from build123d import *

# Parameters (mm, degrees)
ESQUISSE1_W             = 8
ESQUISSE1_H             = 20
BOSS_EXTRU_1_DEPTH      = 12
ESQUISSE2_W             = 8
ESQUISSE2_H             = 10
ENL_V_MAT_EXTRU_1_DEPTH = 8
ESQUISSE3_R             = 3
ENL_V_MAT_EXTRU_2_DEPTH = 10
ESQUISSE4_R             = 3
ENL_V_MAT_EXTRU_3_DEPTH = 4


with BuildPart() as part:
    # Esquisse1 → Boss.-Extru.1 (new body)
    with BuildSketch(Plane.XY):
        Rectangle(ESQUISSE1_W, ESQUISSE1_H)
    extrude(amount=BOSS_EXTRU_1_DEPTH)

    # Esquisse2 → Enlèv. mat.-Extru.1 (cut)
    with BuildSketch(Plane.ZY.offset(4)):
        with Locations((8, -5)):
            Rectangle(ESQUISSE2_W, ESQUISSE2_H)
    extrude(amount=-ENL_V_MAT_EXTRU_1_DEPTH, mode=Mode.SUBTRACT)

    # Esquisse3 → Enlèv. mat.-Extru.2 (cut)
    with BuildSketch(Plane.XZ):
        with Locations(Location((0, 8, 0), (0, 0, 270))):
            Circle(ESQUISSE3_R)
    extrude(amount=-ENL_V_MAT_EXTRU_2_DEPTH, mode=Mode.SUBTRACT)

    # Esquisse4 → Enlèv. mat.-Extru.3 (cut)
    with BuildSketch(Plane.XY.offset(4)):
        with Locations((0, -5)):
            Circle(ESQUISSE4_R)
    extrude(amount=-ENL_V_MAT_EXTRU_3_DEPTH, mode=Mode.SUBTRACT)


solid = part.part
Model file for the job. Use its own axes, mm. A direction names the side the tool comes from. Give positions to 0.01 mm unless a question says otherwise; leave off trailing zeros. Order: outer loops, then holes, each group sorted by start corner. A loop starts at its lowest first (then second) coordinate and runs counter-clockwise, first axis right, second up. Notation, with made-up numbers: (-6.75, 39) - (31.25, 39) arc R23 cw to (31.25, 60) - close; hole circle Ø8 at (58, 84.5). An arc over 180 degrees is marked (long way). One line per item, written item: value.
Item 1: Pin check, flat tips, straight feed: pin 1 Ø4 at (y, z) = (-3.5, 4.5) entering from +X; pin 2 Ø2 at (x, y) = (3, -5.5) entering from +Z. Stop position of each tip, or through.
Response values:
pin 1: x = 4
pin 2: z = 4
Item 2: Slice it at A-A (z = 8). List the corners of the cut face in (x, y).
Response values:
outline: (-4, 0) - (-3, 0) - (-3, 10) - (-4, 10) - close; (3, 0) - (4, 0) - (4, 10) - (3, 10) - close
Item 3: Wall check: line 1 (X direction, y = 4, z = 8); line 2 (Y direction, x = 3, z = 10); line 3 (Y direction, x = 0, z = 0.9). Give the ranges that are in metal, low to high.
Response values:
line 1: -4 to -3, 3 to 4
line 2: 0 to 10
line 3: -10 to -8, -2 to 10
Item 4: Slice it at C-C (x = 0). List the corners of the cut face in (y, z).
Response values:
outline: (-10, 0) - (-8, 0) - (-8, 4) - (-10, 4) - close; (-2, 0) - (10, 0) - (10, 5) - (0, 5) - (0, 4) - (-2, 4) - close; (0, 11) - (10, 11) - (10, 12) - (0, 12) - close
Item 5: Tool access for faces 1 (the flat face through (-3, 0, 10)), 2 (the flat face through (-0.1, 10, 4.6)): list every direction of +Z, -Z, +X, -X, +Y, -Y with a clear straight run to the whole face (end or side of a thin tool).
Response values:
face 1: +Z, +X, -X, -Y
face 2: +Z, -Z, +X, -X, +Y
Item 6: Slice it at B-B (y = -5). List the corners of the cut face in (x, z), then the cut area to 3 significant figures.
Response values:
outline: (-4, 0) - (-3, 0) - (-3, 4) - (-4, 4) - close; (3, 0) - (4, 0) - (4, 4) - (3, 4) - close
area: 8.00 mm2
Item 7: Two-plate mould, pull along Y, no slides. Class faces 3 (the flat face through (0, -10, 2)), 4 (the cylindrical face through (0.9, 4.93, 5.14)), 5 (the cylindrical face through (0, -2, 2)): released by +Y, released by -Y, zero draft, split by the parting line, or undercut.
Response values:
face 3: released by -Y
face 4: zero draft
face 5: undercut
Item 8: Slice it at D-D (y = 1). List the corners of the cut face in (x, z).
Response values:
outline: (-4, 0) - (4, 0) - (4, 12) - (-4, 12) - close; hole circle Ø6 at (0, 8)
